```python
from build123d import *

# Parameters (mm, degrees)
F0_R     = 12.7
F1_DEPTH = 60.325


with BuildPart() as f1:
    # F0 (on Front) → F1 (new body)
    with BuildSketch(Plane.XZ):
        with BuildLine():
            Line((186.3344, 0), (22.352, 0))
            ThreePointArc((22.352, 0), (-15.805251, 15.805251), (0, -22.352))
            Line((0, -22.352), (194.2084, -22.352))
            Line((194.2084, -22.352), (194.2084, -7.874))
            ThreePointArc((194.2084, -7.874), (191.902159, -2.306241), (186.3344, 0))
        make_face()
        Circle(F0_R, mode=Mode.SUBTRACT)
    extrude(amount=F1_DEPTH)


solid = f1.part
```
CAD build for the part. Positions are in the model's coordinates, mm. A direction names the side the tool comes from. Round coordinates to 2 decimals unless told otherwise and drop trailing zeros. Write each loop counter-clockwise with the first axis right and the second up, starting at its lowest first coordinate (ties: lowest second). Pieces come first, ordered by that corner, then holes. Notation, with made-up numbers: (28, 3.5) - (67, 3.5) arc R16 ccw to (67, 12.5) - close; hole circle Ø11 at (27.25, -19). An arc over 180 degrees is marked (long way). Write item = value, one per line. Start each with the question number.
Q1. Probe L1, parallel to Z at x = 0, y = -16; L2, parallel to X at y = -52, z = 7.5; L3, parallel to Z at x = 87, y = -41. List the from-to ranges inside material, lowest first. Write a range as from..to.
Q2. Band-saw the part on B-B (z = -2). Give the cut face in (x, y) (3 decimals), then the cut area to 3 significant figures.
Q3. Band-saw the part on C-C (x = 171.5). Give the cut face in (y, z) (3 decimals), then the cut area to 3 significant figures.
Q4. Drop flat-ended pins along their axis: pin 1 (3 mm diameter, centred on y = -31, z = 7.5, fed in from -X); pin 2 (5 mm diameter, centred on x = 155, y = -6, fed in from +Z); pin 3 (12 mm diameter, centred on y = -42.5, z = 3, fed in from +X). Give the stop position or say it passes through.
Q5. Band-saw the part on A-A (y = -54). Give the cut face in (x, z), then the cut area to 3 significant figures.
Q6. Mould opens along Z. For faces 1 (the cylindrical face through (191.963, -29.74, -2.368)), 2 (the flat face through (96, -30, -22.352)), 3 (the cylindrical face through (-2.75, -29.74, -12.4)) say: pulls with the +Z half, pulls with the -Z half, needs draft (parallel to the pull), parting line crosses it, or undercut.
Q7. Band-saw the part on D-D (z = -10.5). Give the cut face in (x, y) (3 decimals), then the cut area to 3 significant figures.
Q8. Which spindle directions (+Z, -Z, +X, -X, +Y, -Y) get a long thin tool onto all of the face, cutting with end or side? Do faces 4 (the cylindrical face through (-15.275, -29.74, 16.318)), 5 (the flat face through (105, -30, 0)). Say none if no direction does.
Answers below:
q1.L1 = -22.35..-12.7, 12.7..22.35
q1.L2 = -21.06..-10.25, 10.25..21.06
q1.L3 = -22.35..0
q2.outline = (-22.262, -60.325) - (-12.542, -60.325) - (-12.542, 0) - (-22.262, 0) - close; (12.542, -60.325) - (191.578, -60.325) - (191.578, 0) - (12.542, 0) - close
q2.area = 11,400 mm2
q3.outline = (-60.325, -22.352) - (0, -22.352) - (0, 0) - (-60.325, 0) - close
q3.area = 1,350 mm2
q4.pin_1 = -21.53
q4.pin_2 = 0
q4.pin_3 = 192.52
q5.outline = (0, -22.35) - (194.21, -22.35) - (194.21, -7.87) arc R7.87 ccw to (186.33, 0) - (22.35, 0) arc R22.35 ccw (long way) to start; hole circle Ø25.4 at (0, 0)
q5.area = 5,000 mm2
q6.face_1 = pulls with the +Z half
q6.face_2 = pulls with the -Z half
q6.face_3 = undercut
q7.outline = (-19.732, -60.325) - (-7.144, -60.325) - (-7.144, 0) - (-19.732, 0) - close; (7.144, -60.325) - (194.208, -60.325) - (194.208, 0) - (7.144, 0) - close
q7.area = 12,000 mm2
q8.face_4 = +Y, -Y
q8.face_5 = +Z, +X, +Y, -Y
